For this review, use the dimensioned drawing (mm, ordinates from the lowest corner) and the shaded views. A direction names the side the tool comes from. Give positions to 0.01 mm unless a question says otherwise; leave off trailing zeros. Loops run counter-clockwise (first coordinate to the right, second up) from the corner with the lowest first, then second, coordinate; pieces in that order, holes last. Notation, with made-up numbers: M 39.5,-18 L 56.5,-18 A23 ccw 56.5,-3 Z; hole C -36,6.25 d7. An arc over 180 degrees is marked long. Use a Markdown table: item, result. Add a question column.
(1) Draft analysis for pull direction Y (two halves, no side actions). For the marked faces 3, 4 and 5, state which applies: pulls with the +Y half, pulls with the -Y half, needs draft (parallel to the pull), parting line crosses it, or undercut.
(2) For probe 1 along X at (y, z) = (10, 4.35); probe 2 along X at (y, z) = (10, 2.85), list the stretches that pass through material, from the lowest coordinate up.
(3) Add section C-C, the plane y = 3. Give the boundary of the cut face in (x, z), then the cut area to 3 significant figures.
(4) For the marked faces 1 and 2, list the 3-axis set-ups (+Z, -Z, +X, -X, +Y, -Y) from which the entire face can be reached by the end or side of a thin tool; tool diameter is ignored.
(5) Add section B-B, the plane z = 4.4. Give the boundary of the cut face in (x, y).
(6) Insertion check: pin 1 Ø1 at (x, y) = (6.5, 16) entering from -Z; pin 2 Ø3 at (x, z) = (5.5, 0.5) entering from -Y; pin 3 Ø0.9 at (x, y) = (3, 10) entering from -Z; pin 4 Ø2.5 at (x, y) = (10, 17) entering from +Z. Each pin has a flat end and moves straight along its axis. Give the tip position at first contact, or say it passes through.
(7) Add section D-D, the plane x = 3.25. Give the boundary of the cut face in (y, z), then the cut area to 3 significant figures.
(8) Add section A-A, the plane y = 10. Give the boundary of the cut face in (x, z), then the cut area to 3 significant figures.
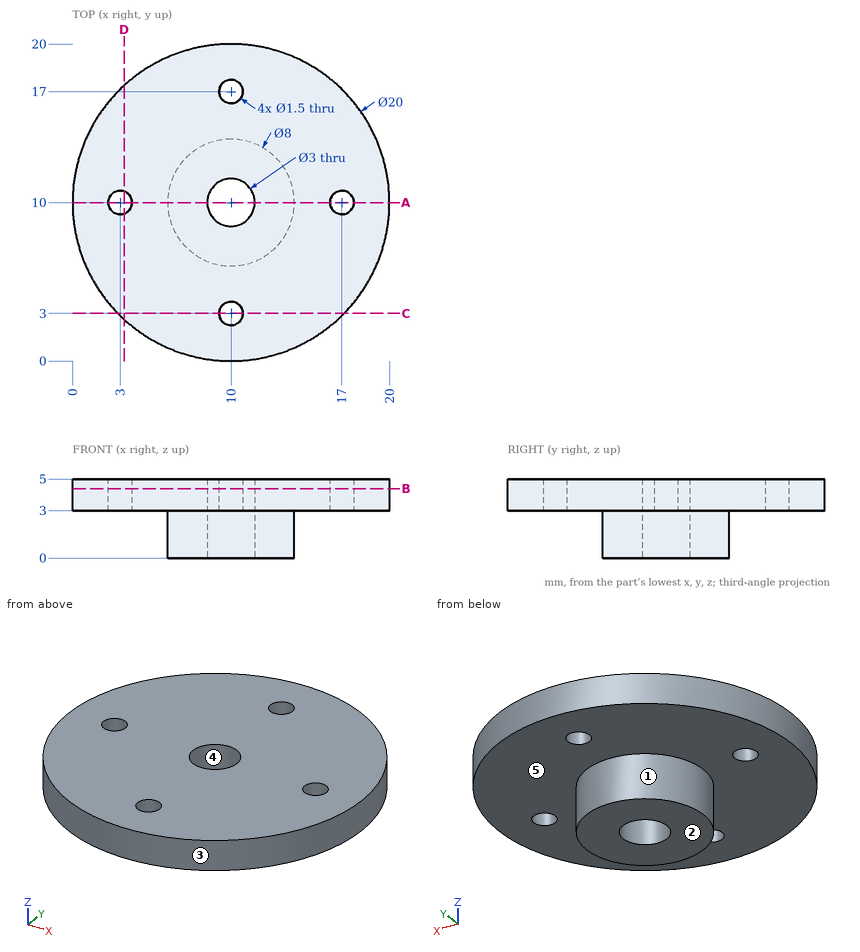
Established:
| question | item | result |
|---|---|---|
| 1 | face 3 | parting line crosses it |
| 1 | face 4 | undercut |
| 1 | face 5 | needs draft |
| 2 | probe 1 | 0 to 2.25, 3.75 to 8.5, 11.5 to 16.25, 17.75 to 20 |
| 2 | probe 2 | 6 to 8.5, 11.5 to 14 |
| 3 | outline | M 2.86,3 L 9.25,3 L 9.25,5 L 2.86,5 Z; M 10.75,3 L 17.14,3 L 17.14,5 L 10.75,5 Z |
| 3 | area | 25.6 mm^2 |
| 4 | face 1 | -Z |
| 4 | face 2 | -Z, +X, -X, +Y, -Y |
| 5 | outline | C 10,10 d20; hole C 3,10 d1.5; hole C 10,10 d3; hole C 10,3 d1.5; hole C 10,17 d1.5; hole C 17,10 d1.5 |
| 6 | pin 1 | z = 3 |
| 6 | pin 2 | y = 7.35 |
| 6 | pin 3 | through |
| 6 | pin 4 | z = 5 |
| 7 | outline | M 2.62,3 L 9.29,3 L 9.29,5 L 2.62,5 Z; M 10.71,3 L 17.38,3 L 17.38,5 L 10.71,5 Z |
| 7 | area | 26.7 mm^2 |
| 8 | outline | M 0,3 L 2.25,3 L 2.25,5 L 0,5 Z; M 3.75,3 L 6,3 L 6,0 L 8.5,0 L 8.5,5 L 3.75,5 Z; M 11.5,0 L 14,0 L 14,3 L 16.25,3 L 16.25,5 L 11.5,5 Z; M 17.75,3 L 20,3 L 20,5 L 17.75,5 Z |
| 8 | area | 43.0 mm^2 |
